Source: CAD feature listing. Evaluate the final solid. Frame: model axes, mm. Round coordinates to 2 decimals unless told otherwise and drop trailing zeros. Order: outer loops, then holes, each group sorted by start corner. A loop starts at its lowest first (then second) coordinate and runs counter-clockwise, first axis right, second up. Notation, with made-up numbers: (37, 65.25) - (43, 65.25) arc R21 cw to (43, 83.25) - close; hole circle Ø11 at (-23, -38). An arc over 180 degrees is marked (long way). Put each result on its own line as item: value. Start each with the question number.
1) Contact query for a flat-ended pin moving along its axis: P1, Ø5.5, axis at x = 0, z = 76, coming from the +Y side. Output: stop coordinate, or through.
2) Section C-C on x = 0. Output: boundary loops of the cut face in (y, z), then the cut area to 3 significant figures.
3) Mould query, pull axis Z, two halves, no side actions, for faces 1 (the face through (-2, 8, -150)), 2 (the face through (-72.45, 7.4, 30.79)), 3 (the face through (-120, 8, -18)). Classes: +Z half, -Z half, draft (parallel to the pull), parting line (faces both ways), or undercut.
4) Line query: probe 1 along X at (y, z) = (10.75, 33); probe 2 along X at (y, z) = (3.75, -96); probe 3 along Z at (x, y) = (72, 11). Output: solid intervals per line, ascending. Write a range as [from, to].
5) Section B-B on z = -53. Output: boundary loops of the cut face in (x, y), then the cut area to 3 significant figures.
6) Section A-A on z = -96. Output: boundary loops of the cut face in (x, y), then the cut area to 3 significant figures.
```python
from build123d import *

# Parameters (mm, degrees)
CROQUIS1_W              = 240
CROQUIS1_H              = 220
CROQUIS1_R              = 3
SALIENTE_EXTRUIR1_DEPTH = 15
CROQUIS2_W              = 240
CROQUIS2_H              = 40
SALIENTE_EXTRUIR2_DEPTH = 15


with BuildPart() as part:
    # Croquis1 → Saliente-Extruir1 (new body)
    with BuildSketch(Plane(origin=(0, 0, 0), x_dir=(1, 0, 0), z_dir=(0, 1, 0))):
        Rectangle(CROQUIS1_W, CROQUIS1_H)
        with Locations(Location((0, 96, 0), (0, 0, 270))):
            Circle(CROQUIS1_R, mode=Mode.SUBTRACT)
        with Locations(Location((0, -76, 0), (0, 0, 270))):
            Circle(CROQUIS1_R, mode=Mode.SUBTRACT)
        with Locations(Location((-74.47818473, 53, 0), (0, 0, 270))):
            Circle(CROQUIS1_R, mode=Mode.SUBTRACT)
        with Locations(Location((-74.47818473, -33, 0), (0, 0, 270))):
            Circle(CROQUIS1_R, mode=Mode.SUBTRACT)
        with Locations(Location((74.47818473, 53, 0), (0, 0, 270))):
            Circle(CROQUIS1_R, mode=Mode.SUBTRACT)
        with Locations(Location((74.47818473, -33, 0), (0, 0, 270))):
            Circle(CROQUIS1_R, mode=Mode.SUBTRACT)
    extrude(amount=SALIENTE_EXTRUIR1_DEPTH)

    # Croquis2 → Saliente-Extruir2 (add)
    with BuildSketch(Plane(origin=(0, 15, 0), x_dir=(1, 0, 0), z_dir=(0, 1, 0))):
        with Locations((0, 130)):
            Rectangle(CROQUIS2_W, CROQUIS2_H)
    extrude(amount=-SALIENTE_EXTRUIR2_DEPTH)


solid = part.part
```
Answer sheet:
1. P1: through
2. outline: (0, -150) - (15, -150) - (15, -99) - (0, -99) - close; (0, -93) - (15, -93) - (15, 73) - (0, 73) - close; (0, 79) - (15, 79) - (15, 110) - (0, 110) - close
2. area: 3,720 mm^2
3. face 1: -Z half
3. face 2: undercut
3. face 3: draft
4. probe 1: [-120, -77.48], [-71.48, 71.48], [77.48, 120]
4. probe 2: [-120, -3], [3, 120]
4. probe 3: [-150, -54.69], [-51.31, 31.31], [34.69, 110]
5. outline: (-120, 0) - (-77.48, 0) - (-77.48, 15) - (-120, 15) - close; (-71.48, 0) - (71.48, 0) - (71.48, 15) - (-71.48, 15) - close; (77.48, 0) - (120, 0) - (120, 15) - (77.48, 15) - close
5. area: 3,420 mm^2
6. outline: (-120, 0) - (-3, 0) - (-3, 15) - (-120, 15) - close; (3, 0) - (120, 0) - (120, 15) - (3, 15) - close
6. area: 3,510 mm^2
